Input: part model. Units: mm. Frame: model coordinates. Round coordinates to 2 decimals unless told otherwise and drop trailing zeros. Loops run counter-clockwise (first coordinate to the right, second up) from the corner with the lowest first, then second, coordinate; pieces in that order, holes last. Notation, with made-up numbers: M 67.5,-7 L 114.5,-7 A25 ccw 114.5,14 Z; hole C -29,55 d1. An arc over 180 degrees is marked long. Use one line per item in the form item = value. Start each with the question number.
Q1. First-contact query: P1, Ø1.5, axis at x = -104.5, z = 3.5, coming from the -Y side; P2, Ø2.5, axis at y = -24.5, z = 2.5, coming from the +X side; P3, Ø4, axis at x = -92, y = 83, coming from the -Z side; P4, Ø1.5, axis at x = 10, z = 1.5, coming from the -Y side. Flat tips, straight axial feed; report the tip coordinate or a pass-through.
Q2. Section query A-A, the plane x = -48. Output: boundary loops of the cut face in (y, z).
Q3. Section query B-B, the plane y = 90.5. Output: boundary loops of the cut face in (x, z).
Q4. Ray query, line 1 along Y through (x, z) = (-49, 4.3); line 2 along Y through (x, z) = (-106.5, 1.7); line 3 along X through (y, z) = (-25.5, 2.4). Return the intervals inside material, ascending.
Q5. Section query C-C, the plane x = 22.5. Output: boundary loops of the cut face in (y, z), and give its area (3 significant figures).
Q6. Section query D-D, the plane z = 2.05. State how many separate pieces and enclosed holes the cut face has, and give its area (3 significant figures).
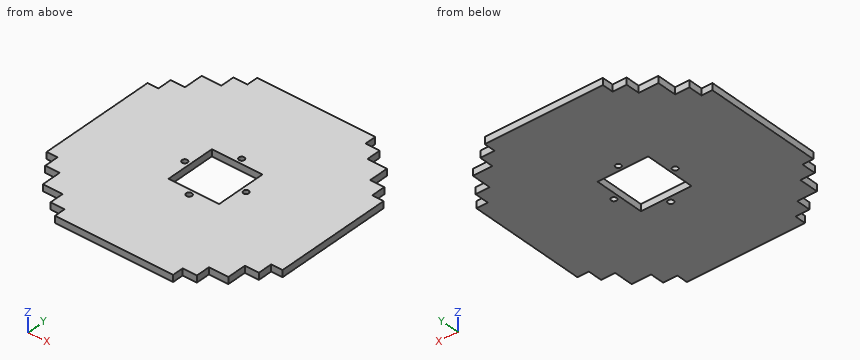
```python
from build123d import *

# Parameters (mm, degrees)
SKETCH1_R           = 2.045707784
SKETCH1_R_2         = 2.13337502
SKETCH1_W           = 38.1
SKETCH1_H           = 38.1
BOSS_EXTRUDE3_DEPTH = 5.08


with BuildPart() as part:
    # Sketch1 → Boss-Extrude3 (new body)
    with BuildSketch(Plane.XY):
        Polygon((-83.014795154, 130.420630372), (5.943060379, 130.420630372), (5.943060379, 121.930337924), (16.626041869, 121.930337924), (16.626041869, 111.260143372), (31.269563819, 111.260143372), (31.269563819, 96.576116387), (41.855511127, 96.576116387), (41.855511127, 85.860143372), (50.436103152, 85.860143372), (50.436103152, -2.997954724), (41.855511127, -2.997954724), (41.855511127, -13.785983185), (31.269563819, -13.785983185), (31.269563819, -28.34797266), (16.626041869, -28.34797266), (16.626041869, -39.015452444), (5.9203896, -39.015452444), (5.9203896, -47.379369628), (-83.037465933, -47.379369628), (-83.037465933, -39.015452444), (-93.601982027, -39.015452444), (-93.601982027, -28.34797266), (-108.414795154, -28.34797266), (-108.414795154, -13.785983185), (-119.192241536, -13.785983185), (-119.192241536, -2.997954724), (-127.363896848, -2.997954724), (-127.363896848, 85.860143372), (-119.192241536, 85.860143372), (-119.192241536, 96.576116387), (-108.414795154, 96.576116387), (-108.414795154, 111.260143372), (-93.601982027, 111.260143372), (-93.601982027, 121.930337924), (-83.014795154, 121.930337924), align=None)
        with Locations((-61.329510567, 41.431094324)):
            Circle(SKETCH1_R, mode=Mode.SUBTRACT)
        with Locations((-38.215510567, 64.545094324)):
            Circle(SKETCH1_R, mode=Mode.SUBTRACT)
        with Locations((-15.101510567, 41.431094324)):
            Circle(SKETCH1_R, mode=Mode.SUBTRACT)
        with Locations((-38.215510567, 18.317094324)):
            Circle(SKETCH1_R_2, mode=Mode.SUBTRACT)
        with Locations((-38.215510567, 41.431094324)):
            Rectangle(SKETCH1_W, SKETCH1_H, mode=Mode.SUBTRACT)
    extrude(amount=BOSS_EXTRUDE3_DEPTH)


solid = part.part
```
Results found:
q1.P1 = -28.35
q1.P2 = 31.27
q1.P3 = 0
q1.P4 = -39.02
q2.outline = M -47.38,0 L 22.38,0 L 22.38,5.08 L -47.38,5.08 Z; M 60.48,0 L 130.42,0 L 130.42,5.08 L 60.48,5.08 Z
q3.outline = M -119.19,0 L 41.86,0 L 41.86,5.08 L -119.19,5.08 Z
q4.line_1 = -47.38 to 22.38, 60.48 to 130.42
q4.line_2 = -28.35 to 111.26
q4.line_3 = -108.41 to 31.27
q5.outline = M -28.35,0 L 111.26,0 L 111.26,5.08 L -28.35,5.08 Z
q5.area = 709 mm²
q6.separate_pieces = 1
q6.enclosed_holes = 5
q6.area = 25,700 mm²
